Could you check a few things on this model? Use its own coordinates, in mm. A direction names the side the tool comes from. Round coordinates to 2 decimals unless told otherwise and drop trailing zeros. Write each question's results on one line, items separated by ' | '. Start each with the question number.
1) Imagine slicing it at A-A, the plane z = 2.05. Give the number of separate pieces and of enclosed holes in the cut face, plus the area to 4 significant figures.
2) We'd pull the mould along X, two halves only. Please class faces 1 (the flat face through (-60.325, -33, 1)), 2 (the flat face through (50.8, 0, 1)), 3 (the flat face through (-74.435, -29, 1)), 4 (the flat face through (-28, -1, 0)): pulls with the +X half, pulls with the -X half, needs draft (parallel to the pull), parting line crosses it, or undercut.
3) If I drill on probe 1 along X at (y, z) = (22.5, 2.85); probe 2 along Y at (x, z) = (-78, 1.2); probe 3 along X at (y, z) = (6, 1.85), over which ranges is the centre line in solid material (lowest first)?
4) For P1, Ø1.5, axis at x = -31, z = 2, coming from the -Y side; P2, Ø0.9, axis at x = -25.5, z = 1, coming from the -Y side; P3, Ø0.9, axis at y = 15, z = 1.5, coming from the -X side; P4, Ø6, axis at x = 21.5, y = -1.5, coming from the -Z side, each with a flat end and sliding along its axis, tell me the tip position at first contact or that it passes through.
5) Which directions (+Z, -Z, +X, -X, +Y, -Y) give clear straight access to the entire face, cutting with the end or side of a thin tool? Please do faces 5 (the flat face through (39, -31.75, 1)), 6 (the flat face through (42.72, 6, 1)), 7 (the flat face through (27.165, -29, 1)).
from build123d import *

# Parameters (mm, degrees)
SKETCH1_W           = 3
SKETCH1_H           = 25.4
SKETCH1_W_2         = 6.35
SKETCH1_H_2         = 3
BOSS_EXTRUDE1_DEPTH = 3


with BuildPart() as part:
    # Sketch1 → Boss-Extrude1 (new body)
    with BuildSketch(Plane.XY):
        with BuildLine():
            Line((-69.423123959, 31.75), (50.8, 31.75))
            Line((50.8, 31.75), (50.8, -31.75))
            Line((50.8, -31.75), (27.1653, -31.75))
            Line((27.1653, -31.75), (27.1653, -26.67))
            Line((27.1653, -26.67), (29.5275, -26.67))
            Line((29.5275, -26.67), (29.5275, -21.59))
            Line((29.5275, -21.59), (21.2725, -21.59))
            Line((21.2725, -21.59), (21.2725, -26.67))
            Line((21.2725, -26.67), (23.6347, -26.67))
            Line((23.6347, -26.67), (23.6347, -31.75))
            Line((23.6347, -31.75), (9.525, -31.75))
            Line((9.525, -31.75), (9.525, -34.75))
            Line((9.525, -34.75), (-9.525, -34.75))
            Line((-9.525, -34.75), (-9.525, -31.75))
            Line((-9.525, -31.75), (-23.6347, -31.75))
            Line((-23.6347, -31.75), (-23.6347, -26.67))
            Line((-23.6347, -26.67), (-21.2725, -26.67))
            Line((-21.2725, -26.67), (-21.2725, -21.59))
            Line((-21.2725, -21.59), (-29.5275, -21.59))
            Line((-29.5275, -21.59), (-29.5275, -26.67))
            Line((-29.5275, -26.67), (-27.1653, -26.67))
            Line((-27.1653, -26.67), (-27.1653, -31.75))
            Line((-27.1653, -31.75), (-41.275, -31.75))
            Line((-41.275, -31.75), (-41.275, -34.75))
            Line((-41.275, -34.75), (-60.325, -34.75))
            Line((-60.325, -34.75), (-60.325, -31.75))
            Line((-60.325, -31.75), (-74.4347, -31.75))
            Line((-74.4347, -31.75), (-74.4347, -26.67))
            Line((-74.4347, -26.67), (-72.0725, -26.67))
            Line((-72.0725, -26.67), (-72.0725, -21.59))
            Line((-72.0725, -21.59), (-80.3275, -21.59))
            Line((-80.3275, -21.59), (-80.3275, -26.67))
            Line((-80.3275, -26.67), (-77.9653, -26.67))
            Line((-77.9653, -26.67), (-77.9653, -31.75))
            Line((-77.9653, -31.75), (-114.3, -31.75))
            add(Edge.make_bspline(
                [(-114.3, -31.75), (-155.075216818, -12.249007941), (-95.203771035, -1.48614813), (-82.940088204, 30.901814597), (-69.423123959, 31.75)],
                knots=[0, 0, 0, 0, 0.663381838, 1, 1, 1, 1], degree=3))
        make_face()
        with BuildLine():
            Line((33.200035124, 19.05), (33.200035124, 6.35))
            ThreePointArc((33.200035124, 6.35), (25.580035124, -1.27), (17.960035124, 6.35))
            Line((17.960035124, 6.35), (17.960035124, 19.05))
            ThreePointArc((17.960035124, 19.05), (25.580035124, 26.67), (33.200035124, 19.05))
        make_face(mode=Mode.SUBTRACT)
        with BuildLine():
            Line((-69.423123959, 0), (-69.423123959, 21.185554356))
            add(Edge.make_bspline(
                [(-69.423123959, 21.185554356), (-77.065116074, 19.019259029), (-89.179513015, 16.560411812), (-97.292708494, 3.952124557), (-94.492767951, 0)],
                knots=[0, 0, 0, 0, 0.649291819, 1, 1, 1, 1], degree=3))
            Line((-94.492767951, 0), (-69.423123959, 0))
        make_face(mode=Mode.SUBTRACT)
        with BuildLine():
            Line((0.180035124, 19.05), (0.180035124, 6.35))
            ThreePointArc((0.180035124, 6.35), (-7.439964876, -1.27), (-15.059964876, 6.35))
            Line((-15.059964876, 6.35), (-15.059964876, 19.05))
            ThreePointArc((-15.059964876, 19.05), (-7.439964876, 26.67), (0.180035124, 19.05))
        make_face(mode=Mode.SUBTRACT)
        with BuildLine():
            Line((-32.839964876, 19.05), (-32.839964876, 6.35))
            ThreePointArc((-32.839964876, 6.35), (-40.459964876, -1.27), (-48.079964876, 6.35))
            Line((-48.079964876, 6.35), (-48.079964876, 19.05))
            ThreePointArc((-48.079964876, 19.05), (-40.459964876, 26.67), (-32.839964876, 19.05))
        make_face(mode=Mode.SUBTRACT)
        with Locations((44.22, 6.35)):
            Rectangle(SKETCH1_W, SKETCH1_H, mode=Mode.SUBTRACT)
        with Locations((-75.2475, 26.052973764)):
            Rectangle(SKETCH1_W_2, SKETCH1_H_2, mode=Mode.SUBTRACT)
    extrude(amount=BOSS_EXTRUDE1_DEPTH)


solid = part.part
Checked values:
1) separate pieces: 1 | enclosed holes: 6 | area: 8,465 mm^2
2) face 1: pulls with the -X half | face 2: pulls with the +X half | face 3: undercut | face 4: needs draft
3) probe 1: -86.41 to -47.25, -33.67 to -14.23, -0.65 to 18.79, 32.37 to 50.8 | probe 2: -31.75 to -26.67, -21.59 to 0, 18.74 to 24.55, 27.55 to 29.44 | probe 3: -103.96 to -95.13, -69.42 to -48.07, -32.85 to -15.05, 0.17 to 17.97, 33.19 to 42.72, 45.72 to 50.8
4) P1: y = -31.75 | P2: y = -21.59 | P3: x = -93.49 | P4: z = 0
5) face 5: +Z, -Z, +X, -Y | face 6: +Z, -Z | face 7: +Z, -Z, -Y
